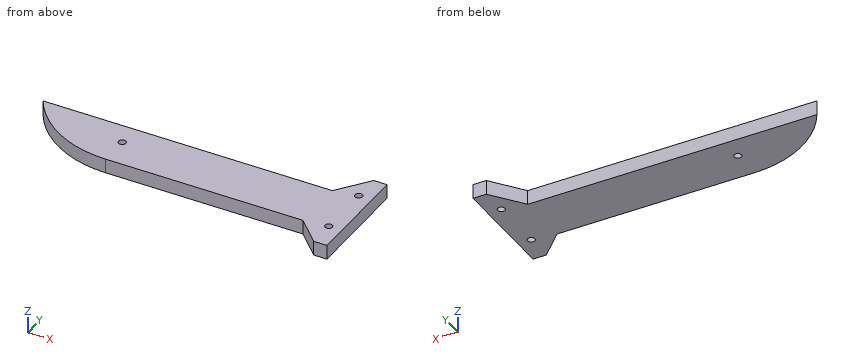
from build123d import *

# Parameters (mm, degrees)
SKETCH1_R           = 1.5
BOSS_EXTRUDE1_DEPTH = 6


with BuildPart() as part:
    # Sketch1 → Boss-Extrude1 (new body)
    with BuildSketch(Plane.XY):
        with BuildLine():
            Line((0, -3), (120, -3))
            Line((120, -3), (130, 10))
            Line((130, 10), (135.5, 10))
            Line((135.5, 10), (135.5, -35))
            Line((135.5, -35), (130, -35))
            Line((130, -35), (120, -25))
            Line((120, -25), (38.105117767, -25))
            ThreePointArc((38.105117767, -25), (16.105117767, -19.105117767), (0, -3))
        make_face()
        with Locations((130, -1.25)):
            Circle(SKETCH1_R, mode=Mode.SUBTRACT)
        with Locations((130, -23.75)):
            Circle(SKETCH1_R, mode=Mode.SUBTRACT)
        with Locations((38.105117767, -12.5)):
            Circle(SKETCH1_R, mode=Mode.SUBTRACT)
    extrude(amount=BOSS_EXTRUDE1_DEPTH)


solid = part.part
Could you check a few things on this model? Use its own coordinates, in mm. Give positions to 0.01 mm unless a question says otherwise; leave off trailing zeros. Order: outer loops, then holes, each group sorted by start corner. A loop starts at its lowest first (then second) coordinate and runs counter-clockwise, first axis right, second up.
1. Suppose I cut it at A-A (z = 2.8). Write out the boundary of the cut face in (x, y), plus the area to 3 significant figures.
Answers below:
outline: (0, -3) arc R44 ccw to (38.11, -25) - (120, -25) - (130, -35) - (135.5, -35) - (135.5, 10) - (130, 10) - (120, -3) - close; hole circle Ø3 at (38.11, -12.5); hole circle Ø3 at (130, -23.75); hole circle Ø3 at (130, -1.25)
area: 2,960 mm2
2. For pin 1 (1.8 mm diameter, centred on x = 38.11, y = -12.5, fed in from +Z); pin 2 (3 mm diameter, centred on x = 30.5, z = 2, fed in from +Y); pin 3 (8 mm diameter, centred on x = 21.5, y = -0.5, fed in from -Z); pin 4 (2 mm diameter, centred on y = 0, z = 2.5, fed in from -X), each with a flat end and sliding along its axis, tell me the tip position at first contact or that it passes through.
Answers below:
pin 1: passes through
pin 2: stops at y = -3
pin 3: stops at z = 0
pin 4: stops at x = 121.54
3. Suppose I cut it at D-D (y = -27.5). Write out the boundary of the cut face in (x, z).
Answers below:
outline: (122.5, 0) - (135.5, 0) - (135.5, 6) - (122.5, 6) - close
4. Suppose I cut it at B-B (y = -1.25). Write out the boundary of the cut face in (x, z).
Answers below:
outline: (121.35, 0) - (128.5, 0) - (128.5, 6) - (121.35, 6) - close; (131.5, 0) - (135.5, 0) - (135.5, 6) - (131.5, 6) - close
5. Suppose I cut it at C-C (x = 94). Write out the boundary of the cut face in (y, z), plus the area to 3 significant figures.
Answers below:
outline: (-25, 0) - (-3, 0) - (-3, 6) - (-25, 6) - close
area: 132 mm2
6. I need wall thicknesses on L1, parallel to Y at x = 130, z = 1.8; L2, parallel to Y at x = 39, z = 4; L3, parallel to X at y = -12, z = 3.8. Which ranges of each line are inside material? Lowest first, please.
Answers below:
L1: y = -35 to -25.25, -22.25 to -2.75, 0.25 to 10
L2: y = -25 to -13.7, -11.3 to -3
L3: x = 6.88 to 36.69, 39.52 to 135.5
